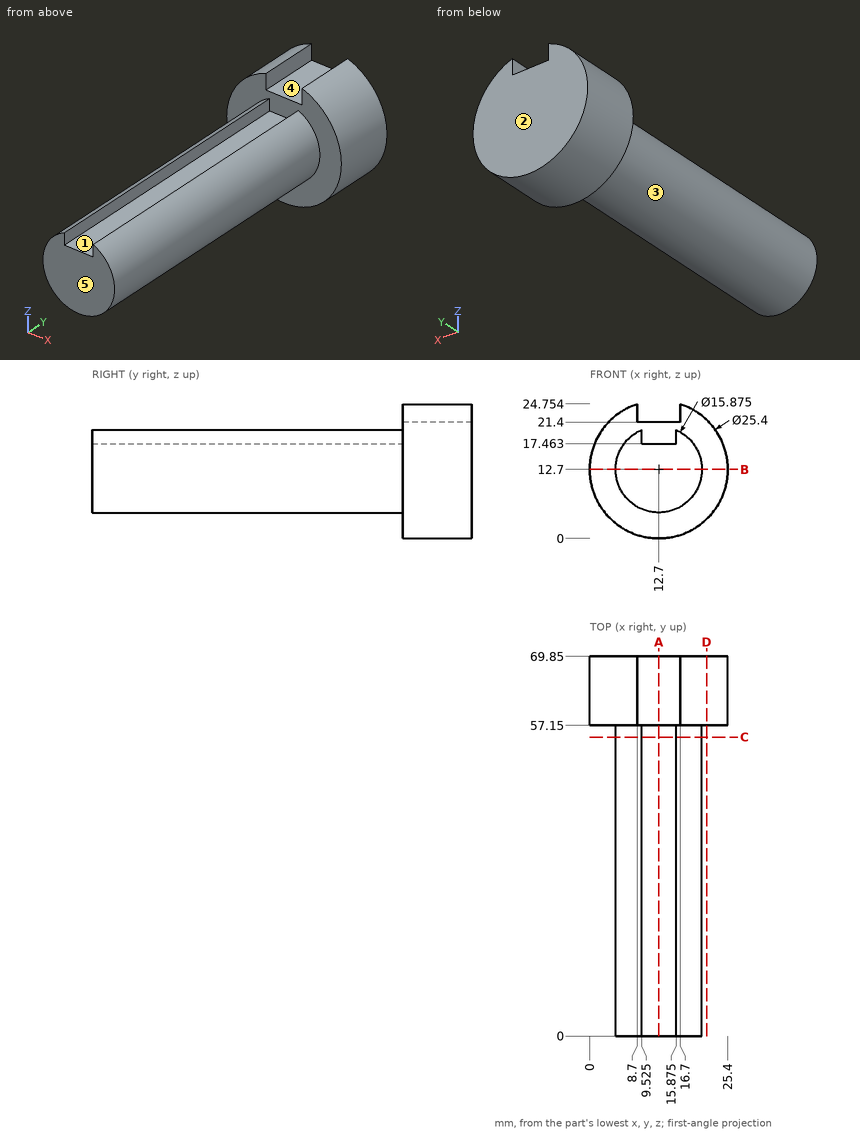
Input: dimensioned drawing with shaded views. Units: mm. Origin: part minimum x, y, z. A direction names the side the tool comes from. Give positions to 0.01 mm unless a question says otherwise; leave off trailing zeros. Write each loop counter-clockwise with the first axis right and the second up, starting at its lowest first coordinate (ties: lowest second). Pieces come first, ordered by that corner, then holes.
1. Draft query along X for the marked faces 1, 2 and 3. Return one class per face: released by +X, released by -X, zero draft, split by the parting line, or undercut.
2. Section query D-D, the plane x = 21.5. Return loops of the section in (y, z).
3. Section query A-A, the plane x = 12.7. Return loops of the section in (y, z).
4. Section query B-B, the plane z = 12.7. Return loops of the section in (x, y), then the cut area to 3 significant figures.
5. Section query C-C, the plane y = 55. Return loops of the section in (x, z) (1 decimal), then the cut area to 3 significant figures.
6. Reachability of the marked faces 4 and 5 from +Z, -Z, +X, -X, +Y, -Y: full face, straight path, thin tool, end or side. Return the list, or none.
7. Pin query (flat end, axial travel): P1, Ø1.3, axis at y = 27.5, z = 18, coming from the -X side; P2, Ø3.5, axis at y = 61, z = 23.5, coming from the -X side; P3, Ø1.5, axis at y = 10, z = 13.5, coming from the -X side. Return the tip coordinate at first contact, or that it passes through.
8. Line query: probe 1 along Y at (x, z) = (4, 12.75); probe 2 along X at (y, z) = (19.5, 12.25) (1 decimal); probe 3 along X at (y, z) = (55, 18.75) (1 decimal). Output: solid intervals per line, ascending.
Computed:
1. face 1: undercut
1. face 2: zero draft
1. face 3: split by the parting line
2. outline: (57.15, 3.54) - (69.85, 3.54) - (69.85, 21.86) - (57.15, 21.86) - close
3. outline: (0, 4.76) - (57.15, 4.76) - (57.15, 0) - (69.85, 0) - (69.85, 21.4) - (57.15, 21.4) - (57.15, 17.46) - (0, 17.46) - close
4. outline: (0, 57.15) - (4.76, 57.15) - (4.76, 0) - (20.64, 0) - (20.64, 57.15) - (25.4, 57.15) - (25.4, 69.85) - (0, 69.85) - close
4. area: 1,230 mm2
5. outline: (9.5, 17.5) - (9.5, 20) arc R7.9 ccw (long way) to (15.9, 20) - (15.9, 17.5) - close
5. area: 179 mm2
6. face 4: +Z, +Y, -Y
6. face 5: +Z, -Z, +X, -X, -Y
7. P1: stops at x = 6.27
7. P2: stops at x = 3.79
7. P3: stops at x = 4.76
8. probe 1: y = 57.15 to 69.85
8. probe 2: x = 4.8 to 20.6
8. probe 3: x = 7.6 to 9.5, 15.9 to 17.8
